Here's how the part is built. I have some questions about the finished solid (model axes, mm). Face numbers are marked on the shaded views. A direction names the side the tool comes from. Coordinates: 2 decimals unless noted, no trailing zeros. Write each loop counter-clockwise with the first axis right and the second up, starting at its lowest first coordinate (ties: lowest second). Pieces come first, ordered by that corner, then holes. Notation, with made-up numbers: (-28.5, -19) -> (10.5, -19) arc R20 ccw to (10.5, -2) -> close; hole circle Ø2 at (-7, 17). An arc over 180 degrees is marked (long way). Use a Markdown table: item, result. Add a question column.
Item 1: Imagine slicing it at C-C, the plane z = 21. Write out the boundary of the cut face in (x, y).
Item 2: Will these pins go through, and if not, where does the flat tip stop? pin 1 Ø20 at (x, y) = (151.5, 52.5) entering from +Z; pin 2 Ø3 at (x, z) = (141, 10.5) entering from +Y; pin 3 Ø2 at (x, z) = (151.5, 9.5) entering from -Y.
Item 3: Imagine slicing it at B-B, the plane x = 142.5. Write out the boundary of the cut face in (y, z), and give its area (3 significant figures).
Item 4: If I drill on line 1 along Y through (x, z) = (108.5, 18.5); line 2 along X through (y, z) = (-42, 16.25); line 3 along Z through (x, y) = (61, 27.5), over which ranges is the centre line in solid material (lowest first)? Write a range as from..to.
Item 5: Imagine slicing it at A-A, the plane y = 54. Write out the boundary of the cut face in (x, z).
Item 6: On a 3-axis mill with a long thin cutter (end or side, diameter ignored), from which of +Z, -Z, +X, -X, +Y, -Y can I reach the whole of each face in a straight line? I mean the marked faces 1, 2 and 3. Say none if no direction works.
Item 7: Imagine slicing it at D-D, the plane y = -42.5. Write out the boundary of the cut face in (x, z).
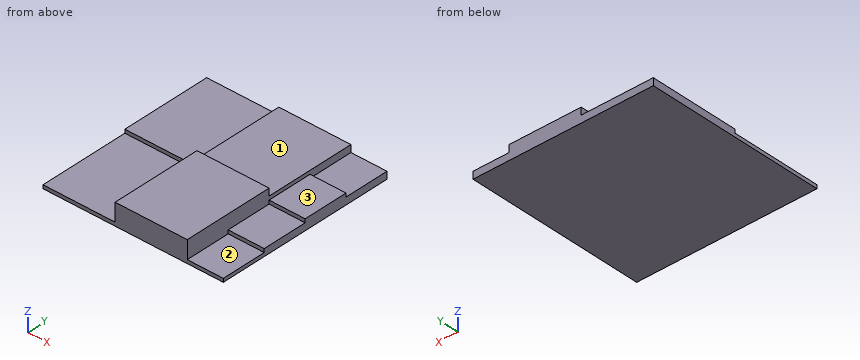
Solid Edge part; units mm, degrees
sketch "Sketch1" plane through (0, 0, 0) normal (0, 0, 1) x (1, 0, 0)
  line L0 (-32.807, 82.2191) -> (-32.807, -17.7809)
  line L1 (-32.807, -17.7809) -> (47.193, -17.7809)
  line L2 (47.193, -17.7809) -> (47.193, 82.2191)
  line L3 (47.193, 82.2191) -> (-32.807, 82.2191)
extrude "Protrusion1" add sketch "Sketch1" along normal blind 8
sketch "Sketch2" plane through (0, 0, 0) normal (0, 0, 1) x (1, 0, 0)
  line L0 (-32.807, -117.7809) -> (-32.807, -17.7809)
  line L1 (-32.807, -17.7809) -> (47.193, -17.7809)
  line L2 (47.193, -17.7809) -> (47.193, -117.7809)
  line L3 (47.193, -117.7809) -> (-32.807, -117.7809)
extrude "ExtrudedProtrusion_2" add sketch "Sketch2" along normal blind 4
sketch "Sketch3" plane through (0, 0, 0) normal (0, 0, 1) x (1, 0, 0)
  line L0 (47.193, 82.2191) -> (127.193, 82.2191)
  line L1 (127.193, 82.2191) -> (127.193, -17.7809)
  line L2 (127.193, -17.7809) -> (47.193, -17.7809)
  line L3 (47.193, -17.7809) -> (47.193, 82.2191)
extrude "ExtrudedProtrusion_3" add sketch "Sketch3" along normal blind 16
sketch "Sketch4" plane through (0, 0, 0) normal (0, 0, 1) x (1, 0, 0)
  line L0 (47.193, -117.7809) -> (127.193, -117.7809)
  line L1 (127.193, -117.7809) -> (127.193, -17.7809)
  line L2 (127.193, -17.7809) -> (47.193, -17.7809)
  line L3 (47.193, -17.7809) -> (47.193, -117.7809)
extrude "ExtrudedProtrusion_4" add sketch "Sketch4" along normal blind 24
sketch "Sketch5" plane through (0, 0, 0) normal (0, 0, 1) x (1, 0, 0)
  line L0 (167.193, -117.7809) -> (127.193, -117.7809)
  line L1 (127.193, -117.7809) -> (127.193, -67.7809)
  line L2 (127.193, -67.7809) -> (167.193, -67.7809)
  line L3 (167.193, -67.7809) -> (167.193, -117.7809)
extrude "ExtrudedProtrusion_5" add sketch "Sketch5" along normal blind 4
sketch "Sketch6" plane through (0, 0, 0) normal (0, 0, 1) x (1, 0, 0)
  line L0 (127.193, -67.7809) -> (167.193, -67.7809)
  line L1 (167.193, -67.7809) -> (167.193, -17.7809)
  line L2 (167.193, -17.7809) -> (127.193, -17.7809)
  line L3 (127.193, -17.7809) -> (127.193, -67.7809)
extrude "ExtrudedProtrusion_6" add sketch "Sketch6" along normal blind 8
sketch "Sketch7" plane through (0, 0, 0) normal (0, 0, 1) x (1, 0, 0)
  line L0 (167.193, -17.7809) -> (127.193, -17.7809)
  line L1 (127.193, -17.7809) -> (127.193, 32.2191)
  line L2 (127.193, 32.2191) -> (167.193, 32.2191)
  line L3 (167.193, 32.2191) -> (167.193, -17.7809)
extrude "ExtrudedProtrusion_7" add sketch "Sketch7" along normal blind 12
sketch "Sketch8" plane through (0, 0, 0) normal (0, 0, 1) x (1, 0, 0)
  line L0 (127.193, 32.2191) -> (167.193, 32.2191)
  line L1 (167.193, 32.2191) -> (167.193, 82.2191)
  line L2 (167.193, 82.2191) -> (127.193, 82.2191)
  line L3 (127.193, 82.2191) -> (127.193, 32.2191)
extrude "ExtrudedProtrusion_8" add sketch "Sketch8" along normal blind 8
Ans:
| question | item | result |
|---|---|---|
| 1 | outline | (47.19, -117.78) -> (127.19, -117.78) -> (127.19, -17.78) -> (47.19, -17.78) -> close |
| 2 | pin 1 | stops at z = 8 |
| 2 | pin 2 | stops at y = 32.22 |
| 2 | pin 3 | stops at y = -17.78 |
| 3 | outline | (-117.78, 0) -> (82.22, 0) -> (82.22, 8) -> (32.22, 8) -> (32.22, 12) -> (-17.78, 12) -> (-17.78, 8) -> (-67.78, 8) -> (-67.78, 4) -> (-117.78, 4) -> close |
| 3 | area | 1,600 mm^2 |
| 4 | line 1 | y = -117.78..-17.78 |
| 4 | line 2 | x = 47.19..127.19 |
| 4 | line 3 | z = 0..16 |
| 5 | outline | (-32.81, 0) -> (167.19, 0) -> (167.19, 8) -> (127.19, 8) -> (127.19, 16) -> (47.19, 16) -> (47.19, 8) -> (-32.81, 8) -> close |
| 6 | face 1 | +Z, +X, -X, +Y |
| 6 | face 2 | +Z, +X, -Y |
| 6 | face 3 | +Z, +X, +Y, -Y |
| 7 | outline | (-32.81, 0) -> (167.19, 0) -> (167.19, 8) -> (127.19, 8) -> (127.19, 24) -> (47.19, 24) -> (47.19, 4) -> (-32.81, 4) -> close |
